Could you check a few things on this model? Use its own coordinates, in mm. A direction names the side the tool comes from. Coordinates: 2 decimals unless noted, no trailing zeros. Order: outer loops, then holes, each group sorted by start corner. A loop starts at its lowest first (then second) coordinate and runs counter-clockwise, first axis right, second up. Notation, with made-up numbers: (-18.5, 14.5) - (-14.5, 14.5) arc R16 cw to (-14.5, 28.5) - close; hole circle Ø10 at (73.5, 82). An arc over 180 degrees is marked (long way). Answer as a JSON object with one key per item and string values. Group by question number.
(1) Will these pins go through, and if not, where does the flat tip stop? P1, Ø6, axis at x = 6, y = -8, coming from the -Z side; P2, Ø0.6, axis at y = -0.5, z = 34, coming from the +X side; P3, Ø8, axis at x = 4.5, z = 7.5, coming from the -Y side; P4, Ø8, axis at y = 4.5, z = 6.5, coming from the +X side.
(2) Imagine slicing it at D-D, the plane z = 31. Write out the boundary of the cut face in (x, y).
(3) Imagine slicing it at B-B, the plane x = 0. Write out the boundary of the cut face in (y, z), and give its area (3 significant figures).
(4) Imagine slicing it at C-C, the plane z = 10. Write out the boundary of the cut face in (x, y).
(5) Please list where these lines run through material, in increasing order: probe 1 along Z at (x, y) = (-6.75, 5); probe 2 along Y at (x, z) = (-0.25, 14.5); probe 3 along X at (y, z) = (-6.5, 14).
(6) Which directions (+Z, -Z, +X, -X, +Y, -Y) give clear straight access to the entire face, cutting with the end or side of a thin tool? Please do faces 1 (the flat face through (-0.994, 0, 34)), 2 (the flat face through (0, 1.124, 34)), 3 (the flat face through (0.994, 0, 34)), 4 (the flat face through (0, -1.124, 34)).
(7) Imagine slicing it at A-A, the plane y = 0. Write out the boundary of the cut face in (x, z), and give its area (3 significant figures).
Autodesk Inventor part; units mm, degrees
ref_plane "YZ Plane" through (0, 0, 0) normal (1, 0, 0) x (0, 1, 0)
ref_plane "XZ Plane" through (0, 0, 0) normal (0, 1, 0) x (-1, 0, 0)
ref_plane "XY Plane" through (0, 0, 0) normal (0, 0, 1) x (1, 0, 0)
sketch "Sketch1" plane through (0, 0, 0) normal (0, 0, 1) x (1, 0, 0)
  circle A0 centre (0, 0) radius 11.5
  dimension "d0" = 23
extrude "Extrusion1" add sketch "Sketch1" along normal blind 30
fillet "Fillet1" radius 3 1 edges at (-11.5, 0, 30)
sketch "Sketch2" plane through (0, 0, 30) normal (0, 0, 1) x (1, 0, 0)
  circle A0 centre (0, 0) radius 1.5
  dimension "d4" = 3
extrude "Extrusion2" add sketch "Sketch2" along normal blind 5
sketch "Sketch3" plane through (0, 0, 35) normal (0, 0, 1) x (1, 0, 0)
  circle A0 centre (0, 0) radius 1.5
  line L0 (-0.9939, -1.1235) -> (0.9939, -1.1235)
  line L1 (0.9939, -1.1235) -> (0.9939, 1.1235)
  line L2 (0.9939, 1.1235) -> (-0.9939, 1.1235)
  line L3 (-0.9939, 1.1235) -> (-0.9939, -1.1235)
  line L4 (-0.9939, -1.1235) -> (0.9939, 1.1235) construction
  line L5 (0.9939, -1.1235) -> (-0.9939, 1.1235) construction
extrude "Extrusion3" cut sketch "Sketch3" against normal blind 2 contours A0 L1 | L2 A0 | A0 L0 | L3 A0
properties part number "Lifting Pad Motor Redo"
Result set:
{
 "1": {"P1": "stops at z = 0", "P2": "stops at x = 0.99", "P3": "stops at y = -11.49", "P4": "stops at x = 11.49"},
 "2": {"outline": "circle Ø3 at (0, 0)"},
 "3": {"outline": "(-11.5, 0) - (11.5, 0) - (11.5, 27) arc R3 ccw to (8.5, 30) - (1.5, 30) - (1.5, 33) - (1.12, 33) - (1.12, 35) - (-1.12, 35) - (-1.12, 33) - (-1.5, 33) - (-1.5, 30) - (-8.5, 30) arc R3 ccw to (-11.5, 27) - close", "area": "700 mm^2"},
 "4": {"outline": "circle Ø23 at (0, 0)"},
 "5": {"probe 1": "z = 0 to 30", "probe 2": "y = -11.5 to 11.5", "probe 3": "x = -9.49 to 9.49"},
 "6": {"face 1": "+Z, -X, +Y, -Y", "face 2": "+Z, +X, -X, +Y", "face 3": "+Z, +X, +Y, -Y", "face 4": "+Z, +X, -X, -Y"},
 "7": {"outline": "(-11.5, 0) - (11.5, 0) - (11.5, 27) arc R3 ccw to (8.5, 30) - (1.5, 30) - (1.5, 33) - (0.99, 33) - (0.99, 35) - (-0.99, 35) - (-0.99, 33) - (-1.5, 33) - (-1.5, 30) - (-8.5, 30) arc R3 ccw to (-11.5, 27) - close", "area": "699 mm^2"}
}
